from build123d import *

# Parameters (mm, degrees)
SKETCH_1_R          = 10
SKETCH_1_R_2        = 1.5
EXTRUDE_1_DEPTH     = 2.5
SKETCH_2_R          = 4.5
EXTRUDE_2_DEPTH     = 2
SKETCH_3_R          = 3
CUT_EXTRUDE_1_DEPTH = 3.5
SKETCH_4_R          = 1.5
CUT_EXTRUDE_2_DEPTH = 3.5


with BuildPart() as part:
    # 草图1 → 凸台-拉伸1 (new body)
    with BuildSketch(Plane.XY):
        Circle(SKETCH_1_R)
        with Locations((0, 7)):
            Circle(SKETCH_1_R_2, mode=Mode.SUBTRACT)
        with Locations((0, -7)):
            Circle(SKETCH_1_R_2, mode=Mode.SUBTRACT)
        with Locations((-7, 0)):
            Circle(SKETCH_1_R_2, mode=Mode.SUBTRACT)
        with Locations((7, 0)):
            Circle(SKETCH_1_R_2, mode=Mode.SUBTRACT)
    extrude(amount=EXTRUDE_1_DEPTH)

    # 草图2 → 凸台-拉伸2 (add)
    with BuildSketch(Plane.XY.offset(2.5)):
        Circle(SKETCH_2_R)
    extrude(amount=EXTRUDE_2_DEPTH)

    # 草图3 → 切除-拉伸1 (cut)
    with BuildSketch(Plane.XY.offset(4.5)):
        Circle(SKETCH_3_R)
    extrude(amount=-CUT_EXTRUDE_1_DEPTH, mode=Mode.SUBTRACT)

    # 草图4 → 切除-拉伸2 (cut)
    with BuildSketch(Plane.XY.offset(1)):
        Circle(SKETCH_4_R)
    extrude(amount=-CUT_EXTRUDE_2_DEPTH, mode=Mode.SUBTRACT)


solid = part.part
Model file for the job. Use its own axes, mm. A direction names the side the tool comes from. Give positions to 0.01 mm unless a question says otherwise; leave off trailing zeros. Loops run counter-clockwise (first coordinate to the right, second up) from the corner with the lowest first, then second, coordinate; pieces in that order, holes last. Notation, with made-up numbers: (-23, 22) -> (6, 22) arc R36 ccw to (6, 57) -> close; hole circle Ø5 at (0, 70). An arc over 180 degrees is marked (long way). Use a Markdown table: item, result. Add a question column.
(1) Tool access for faces 4 (the flat face through (4.3, -2.1, 2.5)), 5 (the cylindrical face through (-0.325, -8.464, 1.232)): list every direction of +Z, -Z, +X, -X, +Y, -Y with a clear straight run to the whole face (end or side of a thin tool).
(2) Wall check: line 1 along X through (y, z) = (1, 0.5); line 2 along Y through (x, z) = (-0.5, 1.75); line 3 along Y through (x, z) = (-0.25, 0.7). Give the ranges that are in metal, low to high.
(3) Mould opens along Y. For faces 1 (the cylindrical face through (-1.5, 0.07, 0.51)), 2 (the cylindrical face through (-0.59, 4.46, 3.49)), 3 (the flat face through (1, -3, 4.5)) say: +Y half, -Y half, draft (parallel to the pull), parting line (faces both ways), or undercut.
(4) Slice it at C-C on z = 1.85. List the corners of the cut face in (x, y), and give its area (3 significant figures).
(5) Slice it at A-A on x = 0. List the corners of the cut face in (y, z), and give its area (3 significant figures).
(6) Slice it at D-D on y = 8.25. List the corners of the cut face in (x, z), and give its area (3 significant figures).
(7) Drop flat-ended pins along their axis: pin 1 Ø2 at (y, z) = (-4, 0.5) entering from -X; pin 2 Ø1.5 at (y, z) = (-2, 0.5) entering from +X. Give the stop position or say it passes through.
Filled sheet:
| question | item | result |
|---|---|---|
| 1 | face 4 | +Z |
| 1 | face 5 | +Z, -Z |
| 2 | line 1 | -9.95 to -8.12, -5.88 to -1.12, 1.12 to 5.88, 8.12 to 9.95 |
| 2 | line 2 | -9.99 to -8.41, -5.59 to -2.96, 2.96 to 5.59, 8.41 to 9.99 |
| 2 | line 3 | -10 to -8.48, -5.52 to -1.48, 1.48 to 5.52, 8.48 to 10 |
| 3 | face 1 | undercut |
| 3 | face 2 | parting line |
| 3 | face 3 | draft |
| 4 | outline | circle Ø20 at (0, 0); hole circle Ø3 at (-7, 0); hole circle Ø6 at (0, 0); hole circle Ø3 at (0, -7); hole circle Ø3 at (0, 7); hole circle Ø3 at (7, 0) |
| 4 | area | 258 mm2 |
| 5 | outline | (-10, 0) -> (-8.5, 0) -> (-8.5, 2.5) -> (-10, 2.5) -> close; (-5.5, 0) -> (-1.5, 0) -> (-1.5, 1) -> (-3, 1) -> (-3, 4.5) -> (-4.5, 4.5) -> (-4.5, 2.5) -> (-5.5, 2.5) -> close; (1.5, 0) -> (5.5, 0) -> (5.5, 2.5) -> (4.5, 2.5) -> (4.5, 4.5) -> (3, 4.5) -> (3, 1) -> (1.5, 1) -> close; (8.5, 0) -> (10, 0) -> (10, 2.5) -> (8.5, 2.5) -> close |
| 5 | area | 29.0 mm2 |
| 6 | outline | (-5.65, 0) -> (-0.83, 0) -> (-0.83, 2.5) -> (-5.65, 2.5) -> close; (0.83, 0) -> (5.65, 0) -> (5.65, 2.5) -> (0.83, 2.5) -> close |
| 6 | area | 24.1 mm2 |
| 7 | pin 1 | x = -9.54 |
| 7 | pin 2 | x = 9.92 |
